Input: part model. Units: mm. Frame: model coordinates. A direction names the side the tool comes from. Round coordinates to 2 decimals unless told otherwise and drop trailing zeros. Loops run counter-clockwise (first coordinate to the right, second up) from the corner with the lowest first, then second, coordinate; pieces in that order, holes last. Notation, with made-up numbers: (70.5, -19.75) -> (124.5, -19.75) arc R25 ccw to (124.5, 4.25) -> close; hole circle Ø5 at (14.25, 83). An arc over 180 degrees is marked (long way). Answer as a JSON object with one key per item and string values.
```python
from build123d import *

# Parameters (mm, degrees)
SKETCH1_R                = 100
BOSS_EXTRUDE2_DEPTH      = 30
BOSS_EXTRUDE2_DEPTH_BACK = 30
SKETCH2_R                = 10
BOSS_EXTRUDE3_DEPTH      = 20
SKETCH3_R                = 10
BOSS_EXTRUDE4_DEPTH      = 20
BOSS_EXTRUDE5_DEPTH      = 4
SKETCH10_W               = 100
SKETCH10_H               = 100
BOSS_EXTRUDE6_DEPTH      = 4


with BuildPart() as part:
    # Sketch1 → Boss-Extrude2 (new body, two sides)
    with BuildSketch(Plane(origin=(0, 0, 0), x_dir=(0, 0, -1), z_dir=(1, 0, 0))) as boss_extrude2_sk:
        Circle(SKETCH1_R)
    extrude(amount=BOSS_EXTRUDE2_DEPTH)
    extrude(boss_extrude2_sk.sketch, amount=-BOSS_EXTRUDE2_DEPTH_BACK)

    # Sketch2 → Boss-Extrude3 (add)
    with BuildSketch(Plane(origin=(30, 0, 0), x_dir=(0, 0, -1), z_dir=(1, 0, 0))):
        Circle(SKETCH2_R)
    extrude(amount=BOSS_EXTRUDE3_DEPTH)

    # Sketch3 → Boss-Extrude4 (add)
    with BuildSketch(Plane.ZY.offset(30)):
        Circle(SKETCH3_R)
    extrude(amount=BOSS_EXTRUDE4_DEPTH)

    # Sketch5 → Boss-Extrude5 (add)
    with BuildSketch(Plane.ZY.offset(50)):
        with BuildLine():
            Line((-17.1736092, -11.211866262), (-115.573756817, 139.51109466))
            ThreePointArc((-115.573756817, 139.51109466), (-109.612013879, 167.896570122), (-81.226538417, 161.934827183))
            Line((-81.226538417, 161.934827183), (17.1736092, 11.211866262))
            ThreePointArc((17.1736092, 11.211866262), (11.211866262, -17.1736092), (-17.1736092, -11.211866262))
        make_face()
    boss_extrude5 = extrude(amount=BOSS_EXTRUDE5_DEPTH)

    # Mirror1: Boss-Extrude5 across plane
    add(boss_extrude5.mirror(Plane(origin=(0, 0, 0), x_dir=(0, 0, 1), z_dir=(1, 0, 0))))

    # Sketch10 → Boss-Extrude6 (add)
    with BuildSketch(Plane(origin=(0, 170, 0), x_dir=(1, 0, 0), z_dir=(0, 1, 0))):
        with Locations((0, 100)):
            Rectangle(SKETCH10_W, SKETCH10_H)
    extrude(amount=BOSS_EXTRUDE6_DEPTH)


solid = part.part
```
1) Draft query along X for faces 1 (the face through (39.86, -9.76, 2.17)), 2 (the face through (-51.97, 63.09, -65.68)), 3 (the face through (-54, 76, -49)). Return one class per face: +X half, -X half, draft (parallel to the pull), parting line (faces both ways), or undercut.
Output:
{"face 1": "undercut", "face 2": "draft", "face 3": "-X half"}
2) Section B-B, the plane y = 144. Output: boundary loops of the cut face in (x, z), plus the area to 3 significant figures.
Output:
{"outline": "(-54, -117.78) -> (-50, -117.78) -> (-50, -69.52) -> (-54, -69.52) -> close; (50, -117.78) -> (54, -117.78) -> (54, -69.52) -> (50, -69.52) -> close", "area": "386 mm^2"}
3) Reachability of faces 4 (the face through (-39.86, -9.76, -2.17)), 5 (the face through (-51.972, 167.646, -109.987)), 6 (the face through (51.972, 87.628, -32.715)), 7 (the face through (51.972, 167.646, -109.987)), 8 (the face through (51.97, 63.09, -65.68)) from +Z, -Z, +X, -X, +Y, -Y: full face, straight path, thin tool, end or side. Return the list, or none.
Output:
{"face 4": "none", "face 5": "-X", "face 6": "+Z, +X, +Y", "face 7": "+X", "face 8": "-Z, +X, -Y"}
4) Section A-A, the plane x = -7. Output: boundary loops of the cut face in (y, z).
Output:
{"outline": "circle Ø200 at (0, 0); (170, -150) -> (174, -150) -> (174, -50) -> (170, -50) -> close"}
5) Section D-D, the plane z = 0. Output: boundary loops of the cut face in (x, y), plus the area to 3 significant figures.
Output:
{"outline": "(-54, -20.51) -> (-50, -20.51) -> (-50, -10) -> (-30, -10) -> (-30, -100) -> (30, -100) -> (30, -10) -> (50, -10) -> (50, -20.51) -> (54, -20.51) -> (54, 37.52) -> (50, 37.52) -> (50, 10) -> (30, 10) -> (30, 100) -> (-30, 100) -> (-30, 10) -> (-50, 10) -> (-50, 37.52) -> (-54, 37.52) -> close", "area": "13,300 mm^2"}
6) Ray query, probe 1 along X at (y, z) = (25, 1); probe 2 along X at (y, z) = (151, -89); probe 3 along X at (y, z) = (66.5, -69.5). Return the intervals inside material, ascending.
Output:
{"probe 1": "x = -54 to -50, -30 to 30, 50 to 54", "probe 2": "x = -54 to -50, 50 to 54", "probe 3": "x = -30 to 30"}
7) Contact query for flat-ended pins moving along their axis: P1, Ø6, axis at x = -12.5, y = -5, coming from the +Z side; P2, Ø5, axis at y = -21, z = -60, coming from the +X side; P3, Ø4.5, axis at y = 172.5, z = -89, coming from the +X side. Output: stop coordinate, or through.
Output:
{"P1": "stops at z = 99.98", "P2": "stops at x = 30", "P3": "stops at x = 50"}
8) Section C-C, the plane x = -46.5. Output: boundary loops of the cut face in (y, z).
Output:
{"outline": "circle Ø20 at (0, 0); (170, -150) -> (174, -150) -> (174, -50) -> (170, -50) -> close"}
